from build123d import *

# Parameters (mm, degrees)
CYLINDER006_R     = 1.15
CYLINDER006_DEPTH = 40
BOX010_W          = 61
BOX010_H          = 61
BOX010_DEPTH      = 7.5
FILLET002_R       = 30


with BuildPart() as obj1:
    # Cylinder006 → Cylinder006 (new body)
    with BuildSketch(Plane(origin=(41, 41, -20), x_dir=(1, 0, 0), z_dir=(0, 0, 1))):
        Circle(CYLINDER006_R)
    extrude(amount=CYLINDER006_DEPTH)


with BuildPart() as cut009:
    # Box010 → Box010 (new body)
    with BuildSketch(Plane.XY.offset(-7.5)):
        with Locations((30.5, 30.5)):
            Rectangle(BOX010_W, BOX010_H)
    extrude(amount=BOX010_DEPTH)

    # Fillet002
    fillet002_edges = [cut009.edges().sort_by_distance(p)[0] for p in [
        (61, 61, -3.75),
    ]]
    fillet(fillet002_edges, radius=FILLET002_R)

    # Cut009: cut obj1
    add(obj1.part, mode=Mode.SUBTRACT)


solid = cut009.part
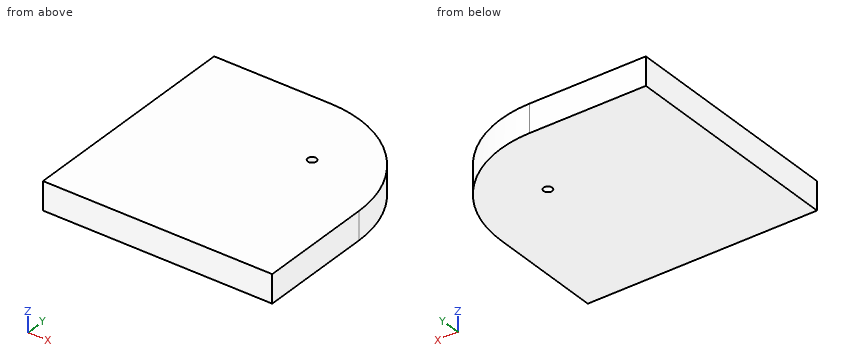
Design review of the part built by this model. Coordinates are the model's own, in mm. Give positions to 0.01 mm unless a question says otherwise; leave off trailing zeros. Write each loop counter-clockwise with the first axis right and the second up, starting at its lowest first coordinate (ties: lowest second). Pieces come first, ordered by that corner, then holes. Notation, with made-up numbers: M 75,32 L 107,32 A16 ccw 107,36 Z; hole C 89.5,13.25 d8. An arc over 180 degrees is marked long. Answer as a JSON object with one key per item and string values. Group by question number.
1) For line 1 along Y through (x, z) = (41, -4); line 2 along X through (y, z) = (57.5, -3), list the stretches that pass through material, from the lowest coordinate up.
2) We need section A-A (y = 41). Give the boundary of the cut face in (x, z), and give its area (3 significant figures).
3) We need section D-D (y = 55.5). Give the boundary of the cut face in (x, z), and give its area (3 significant figures).
4) Clearance check with a flat-ended pin moving along its axis: pin 1 Ø2 at (y, z) = (8, -3.5) entering from -X. State where the tip first meets the part, or that it passes through.
5) We need section C-C (z = -5.5). Give the boundary of the cut face in (x, y), and give its area (3 significant figures).
Answer key:
{
 "1": {"line 1": "y = 0 to 39.85, 42.15 to 59.28", "line 2": "x = 0 to 45.06"},
 "2": {"outline": "M 0,-7.5 L 39.85,-7.5 L 39.85,0 L 0,0 Z; M 42.15,-7.5 L 59.28,-7.5 L 59.28,0 L 42.15,0 Z", "area": "427 mm²"},
 "3": {"outline": "M 0,-7.5 L 48.31,-7.5 L 48.31,0 L 0,0 Z", "area": "362 mm²"},
 "4": {"pin 1": "stops at x = 0"},
 "5": {"outline": "M 0,0 L 61,0 L 61,31 A30 ccw 31,61 L 0,61 Z; hole C 41,41 d2.3", "area": "3,520 mm²"}
}
